from build123d import *
from build123d.topology import SkipClean

# Parameters (mm, degrees)
SKETCH_1_R          = 2.1
EXTRUDE_1_DEPTH     = 5
SKETCH_2_W          = 20
SKETCH_2_H          = 20
SKETCH_2_R          = 2.6
EXTRUDE_2_DEPTH     = 6
SKETCH_3_R          = 5
CUT_EXTRUDE_1_DEPTH = 3
SKETCH_5_W          = 20
SKETCH_5_H          = 20
SKETCH_5_R          = 2.6
EXTRUDE_3_DEPTH     = 6
SKETCH_6_R          = 5
CUT_EXTRUDE_2_DEPTH = 3
SKETCH_7_W          = 20
SKETCH_7_H          = 20
SKETCH_7_R          = 2.6
EXTRUDE_4_DEPTH     = 6
SKETCH_8_R          = 5
CUT_EXTRUDE_3_DEPTH = 3
EXTRUDE_START       = 7.6
SKETCH_9_R          = 5
SKETCH_9_R_2        = 2.1
EXTRUDE_5_DEPTH     = 7.6
EXTRUDE_START_2     = 2.5
SKETCH_10_R         = 5
SKETCH_10_R_2       = 3.95
EXTRUDE_6_DEPTH     = 2.5


with BuildPart() as part:
    # 草图1 → 凸台-拉伸1 (new body)
    with BuildSketch(Plane(origin=(0, 0, 0), x_dir=(1, 0, 0), z_dir=(0, 1, 0))):
        Polygon((0, -65), (0, -130), (150, -130), (150, -65), (85, -65), (85, -20), (32.5, -20), (32.5, -65), align=None)
        with Locations(Location((47.5, -27.5, 0), (0, 0, 270))):
            Circle(SKETCH_1_R, mode=Mode.SUBTRACT)
        with Locations(Location((47.5, -102.5, 0), (0, 0, 270))):
            Circle(SKETCH_1_R, mode=Mode.SUBTRACT)
        with Locations(Location((122.5, -102.5, 0), (0, 0, 270))):
            Circle(SKETCH_1_R, mode=Mode.SUBTRACT)
    extrude(amount=EXTRUDE_1_DEPTH)

    # 草图2 → 凸台-拉伸2 (add)
    with BuildSketch(Plane(origin=(150, 0, 0), x_dir=(0, 0, -1), z_dir=(1, 0, 0))):
        with Locations((-75, -5)):
            Rectangle(SKETCH_2_W, SKETCH_2_H)
        with Locations((-75, -5)):
            Circle(SKETCH_2_R, mode=Mode.SUBTRACT)
    extrude(amount=-EXTRUDE_2_DEPTH)

    # 草图3 → 切除-拉伸1 (cut)
    with BuildSketch(Plane.ZY.offset(-144)):
        with Locations((75, -5)):
            Circle(SKETCH_3_R)
    extrude(amount=-CUT_EXTRUDE_1_DEPTH, mode=Mode.SUBTRACT)

    # 草图5 → 凸台-拉伸3 (add)
    with BuildSketch(Plane(origin=(0, 0, 20), x_dir=(-1, 0, 0), z_dir=(0, 0, -1))):
        with Locations((-75, -5)):
            Rectangle(SKETCH_5_W, SKETCH_5_H)
        with Locations((-75, -5)):
            Circle(SKETCH_5_R, mode=Mode.SUBTRACT)
    extrude(amount=-EXTRUDE_3_DEPTH)

    # 草图6 → 切除-拉伸2 (cut)
    with BuildSketch(Plane.XY.offset(26)):
        with Locations((75, -5)):
            Circle(SKETCH_6_R)
    extrude(amount=-CUT_EXTRUDE_2_DEPTH, mode=Mode.SUBTRACT)

    # 草图7 → 凸台-拉伸4 (add)
    with BuildSketch(Plane(origin=(150, 0, 0), x_dir=(0, 0, -1), z_dir=(1, 0, 0))):
        with Locations((-120, -5)):
            Rectangle(SKETCH_7_W, SKETCH_7_H)
        with Locations((-120, -5)):
            Circle(SKETCH_7_R, mode=Mode.SUBTRACT)
    extrude(amount=-EXTRUDE_4_DEPTH)

    # 草图8 → 切除-拉伸3 (cut)
    with BuildSketch(Plane.ZY.offset(-144)):
        with Locations((120, -5)):
            Circle(SKETCH_8_R)
    extrude(amount=-CUT_EXTRUDE_3_DEPTH, mode=Mode.SUBTRACT)

    # 草图9 → 凸台-拉伸5 (add)
    # profile 1 of 3: a face of its own
    with SkipClean():  # the faces are left unmerged after this step: merging them gives an invalid solid
        with BuildSketch(Plane.XZ.offset(EXTRUDE_START)):
            with Locations(Location((47.5, 102.5, 0), (0, 0, 90))):
                Circle(SKETCH_9_R)
            with Locations(Location((47.5, 102.5, 0), (0, 0, 270))):
                Circle(SKETCH_9_R_2, mode=Mode.SUBTRACT)
        # profile 2 of 3: a face of its own
        with BuildSketch(Plane.XZ.offset(EXTRUDE_START)):
            with Locations(Location((122.5, 102.5, 0), (0, 0, 90))):
                Circle(SKETCH_9_R)
            with Locations(Location((122.5, 102.5, 0), (0, 0, 270))):
                Circle(SKETCH_9_R_2, mode=Mode.SUBTRACT)
        # profile 3 of 3: a face of its own
        with BuildSketch(Plane.XZ.offset(EXTRUDE_START)):
            with Locations(Location((47.5, 27.5, 0), (0, 0, 90))):
                Circle(SKETCH_9_R)
            with Locations(Location((47.5, 27.5, 0), (0, 0, 270))):
                Circle(SKETCH_9_R_2, mode=Mode.SUBTRACT)
        extrude(amount=-EXTRUDE_5_DEPTH)

    # 草图10 → 凸台-拉伸6 (add)
    # profile 1 of 3: a face of its own
    with SkipClean():  # the faces are left unmerged after this step: merging them gives an invalid solid
        with BuildSketch(Plane.XZ.offset(7.6).offset(EXTRUDE_START_2)):
            with Locations(Location((47.5, 102.5, 0), (0, 0, 90))):
                Circle(SKETCH_10_R)
            with Locations(Location((47.5, 102.5, 0), (0, 0, 270))):
                Circle(SKETCH_10_R_2, mode=Mode.SUBTRACT)
        # profile 2 of 3: a face of its own
        with BuildSketch(Plane.XZ.offset(7.6).offset(EXTRUDE_START_2)):
            with Locations(Location((47.5, 27.5, 0), (0, 0, 90))):
                Circle(SKETCH_10_R)
            with Locations(Location((47.5, 27.5, 0), (0, 0, 270))):
                Circle(SKETCH_10_R_2, mode=Mode.SUBTRACT)
        # profile 3 of 3: a face of its own
        with BuildSketch(Plane.XZ.offset(7.6).offset(EXTRUDE_START_2)):
            with Locations(Location((122.5, 102.5, 0), (0, 0, 90))):
                Circle(SKETCH_10_R)
            with Locations(Location((122.5, 102.5, 0), (0, 0, 270))):
                Circle(SKETCH_10_R_2, mode=Mode.SUBTRACT)
        extrude(amount=-EXTRUDE_6_DEPTH)


solid = part.part
Can you work these out from the model? Positions are in its coordinate system, mm. A direction names the side the tool comes from. Round coordinates to 2 decimals unless told otherwise and drop trailing zeros. Loops run counter-clockwise (first coordinate to the right, second up) from the corner with the lowest first, then second, coordinate; pieces in that order, holes last. Notation, with made-up numbers: (86.25, -21) - (142.25, -21) arc R12 ccw to (142.25, -13) - close; hole circle Ø2 at (28.25, 61). An arc over 180 degrees is marked (long way). Answer in a Markdown table with one row per item. Add a question column.
Q1. I want a section at A-A on y = -12. List the corners of the cut face in (x, z) for me.
Q2. I want a section at D-D on y = 3. List the corners of the cut face in (x, z) for me.
Q3. For pin 1 Ø8 at (x, z) = (48.5, 101) entering from -Y; pin 2 Ø4.5 at (y, z) = (-5, 75) entering from -X; pin 3 Ø4 at (x, y) = (24, 2) entering from -Z; pin 4 Ø6 at (x, y) = (115, -3.5) entering from -Z, each with a flat end and sliding along its axis, tell me the tip position at first contact or that it passes through.
Q4. We'd pull the mould along Z, two halves only. Please class faces 1 (the flat face through (144, -11, 120)), 2 (the cylindrical face through (124.415, -5.121, 107.119)), 3 (the cylindrical face through (44.121, -5.121, 23.815)): pulls with the +Z half, pulls with the -Z half, needs draft (parallel to the pull), parting line crosses it, or undercut.
Q5. I want a section at B-B on x = 122.5. List the corners of the cut face in (y, z) for me, and give its area (3 significant figures).
Q6. I need wall thicknesses on L1, parallel to X at y = -8.95, z = 102.5; L2, parallel to Z at x = 122.5, y = -2; L3, parallel to X at y = 3.45, z = 102.5. Which ranges of each line are inside material? Lowest first, please.
Q7. Which directions (+Z, -Z, +X, -X, +Y, -Y) give clear straight access to the entire face, cutting with the end or side of a thin tool? Please do faces 4 (the flat face through (65, -8, 23)), 5 (the flat face through (147, -8, 85)), 6 (the flat face through (85, 1, 37)), 7 (the cylindrical face through (79.619, -6.915, 24.521)), 8 (the cylindrical face through (51.416, -8.868, 28.014)).
A:
| question | item | result |
|---|---|---|
| 1 | outline | (65, 20) - (85, 20) - (85, 26) - (65, 26) - close; (144, 65) - (150, 65) - (150, 85) - (144, 85) - close; (144, 110) - (150, 110) - (150, 130) - (144, 130) - close |
| 2 | outline | (0, 65) - (32.5, 65) - (32.5, 20) - (85, 20) - (85, 65) - (150, 65) - (150, 130) - (0, 130) - close; hole circle Ø4.2 at (47.5, 27.5); hole circle Ø4.2 at (47.5, 102.5); hole circle Ø4.2 at (122.5, 102.5) |
| 3 | pin 1 | y = -10.1 |
| 3 | pin 2 | through |
| 3 | pin 3 | z = 65 |
| 3 | pin 4 | z = 100.32 |
| 4 | face 1 | needs draft |
| 4 | face 2 | parting line crosses it |
| 4 | face 3 | undercut |
| 5 | outline | (-10.1, 97.5) - (0, 97.5) - (0, 65) - (5, 65) - (5, 100.4) - (-7.6, 100.4) - (-7.6, 98.55) - (-10.1, 98.55) - close; (-10.1, 106.45) - (-7.6, 106.45) - (-7.6, 104.6) - (5, 104.6) - (5, 130) - (0, 130) - (0, 107.5) - (-10.1, 107.5) - close |
| 5 | area | 353 mm^2 |
| 6 | L1 | 42.5 to 43.55, 51.45 to 52.5, 117.5 to 118.55, 126.45 to 127.5 |
| 6 | L2 | 97.5 to 100.4, 104.6 to 107.5 |
| 6 | L3 | 0 to 45.4, 49.6 to 120.4, 124.6 to 150 |
| 7 | face 4 | +Z, -Z, -Y |
| 7 | face 5 | +X, -X, -Y |
| 7 | face 6 | -Z, +X, +Y, -Y |
| 7 | face 7 | +Z |
| 7 | face 8 | -Y |
